Geometry: final body of the model. Coordinates: model frame, mm. A direction names the side the tool comes from. Give positions to 0.01 mm unless a question says otherwise; leave off trailing zeros. Order: outer loops, then holes, each group sorted by start corner. A loop starts at its lowest first (then second) coordinate and runs counter-clockwise, first axis right, second up. Notation, with made-up numbers: (21.5, 13) - (52.5, 13) arc R19 cw to (52.5, 31) - close; hole circle Ø11 at (-36, 27). An arc over 180 degrees is marked (long way). Put each result on its own line as item: value. Start each with the question number.
1. Section A-A on z = 19.5. Return the cut outline in (x, y).
2. Ray query, line 1 along Y through (x, z) = (-5, 44.5); line 2 along Z through (x, y) = (-22.5, -33.5). Return the intervals inside material, ascending. Write a range as from..to.
3. Section B-B on x = 13. Return the cut outline in (y, z), plus the area to 3 significant figures.
4. Mould query, pull axis X, two halves, no side actions, for faces 1 (the flat face through (55, -1, 47)), 2 (the flat face through (-1, 50, 49)), 3 (the flat face through (50, -1, 49)), 4 (the flat face through (-1, -55, 47)). Classes: pulls with the +X half, pulls with the -X half, needs draft (parallel to the pull), parting line crosses it, or undercut.
5. Set-up query: faces 5 (the flat face through (-1, 55, 47)), 6 (the flat face through (-1, -50, 49)). Return all of +Z, -Z, +X, -X, +Y, -Y with unobstructed straight access to the full face (end or side cutting, diameter ignored); none if empty.
from build123d import *

# Parameters (mm, degrees)
F0_W     = 100
F0_H     = 100
F1_DEPTH = 100
F2_T     = 5


with BuildPart() as f1:
    # F0 (on Top) → F1 (new body)
    with BuildSketch(Plane.XY):
        Rectangle(F0_W, F0_H)
    extrude(amount=F1_DEPTH)

    # F2
    f2_openings = [f1.faces().sort_by_distance(p)[0] for p in [
        (0, 0, 100),
    ]]
    offset(amount=F2_T, openings=f2_openings, kind=Kind.INTERSECTION)


solid = f1.part
Resolved:
1. outline: (-55, -55) - (55, -55) - (55, 55) - (-55, 55) - close; hole (-50, -50) - (50, -50) - (50, 50) - (-50, 50) - close
2. line 1: -55..-50, 50..55
2. line 2: -5..0
3. outline: (-55, -5) - (55, -5) - (55, 100) - (50, 100) - (50, 0) - (-50, 0) - (-50, 100) - (-55, 100) - close
3. area: 1,550 mm^2
4. face 1: pulls with the +X half
4. face 2: undercut
4. face 3: undercut
4. face 4: needs draft
5. face 5: +Z, -Z, +X, -X, +Y
5. face 6: +Z
